Print and shaded views of the part. All mm, measured from the part's lowest x, y and z. A direction names the side the tool comes from. Coordinates: 2 decimals unless noted, no trailing zeros. Loops run counter-clockwise (first coordinate to the right, second up) from the corner with the lowest first, then second, coordinate; pieces in that order, holes last. Notation, with made-up numbers: M 60,1.25 L 79,1.25 A14 cw 79,8.25 Z; hole C 72,-7.75 d4. An arc over 180 degrees is marked long. Use a Markdown table: item, result. Add a question column.
1) Pin check, flat tips, straight feed: pin 1 Ø3 at (y, z) = (8.5, 92) entering from -X; pin 2 Ø3 at (y, z) = (9.5, 87.5) entering from -X; pin 3 Ø6 at (x, z) = (7, 98) entering from -Y. Stop position of each tip, or through.
2) Band-saw the part on C-C (z = 15). List the corners of the cut face in (x, y) (1 decimal).
3) Band-saw the part on A-A (x = 6.75). List the corners of the cut face in (y, z), plus the area to 3 significant figures.
4) Band-saw the part on B-B (y = 8.5). List the corners of the cut face in (x, z) (1 decimal).
5) Wall check: probe 1 along Z at (x, y) = (3.25, 1.75); probe 2 along Y at (x, z) = (7, 19.5); probe 3 along X at (y, z) = (8.25, 102.5). Give the ranges that are in metal, low to high. Write a range as from..to.
6) Band-saw the part on D-D (x = 12.5). List the corners of the cut face in (y, z), plus the area to 3 significant figures.
7) Tool access for the marked faces 1 and 2: list every direction of +Z, -Z, +X, -X, +Y, -Y with a clear straight run to the whole face (end or side of a thin tool).
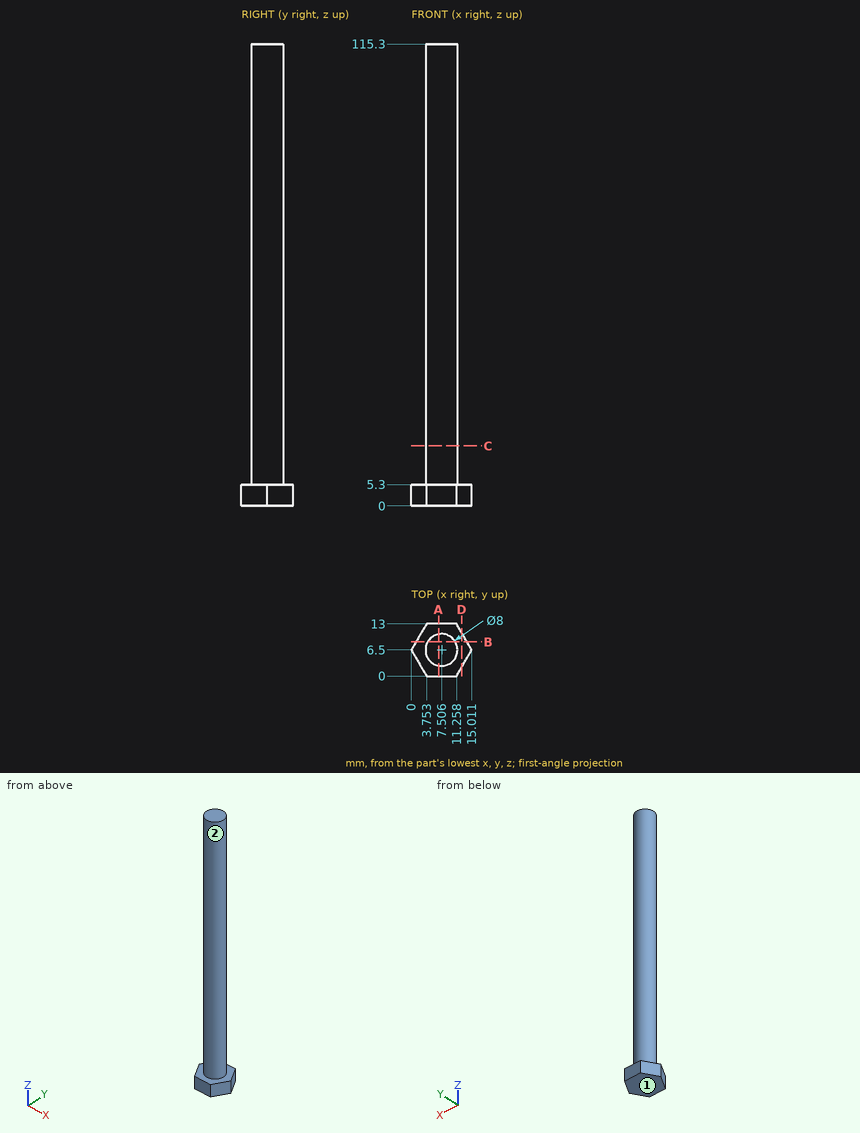
Entries:
| question | item | result |
|---|---|---|
| 1 | pin 1 | x = 3.54 |
| 1 | pin 2 | x = 3.8 |
| 1 | pin 3 | y = 2.5 |
| 2 | outline | C 7.5,6.5 d8 |
| 3 | outline | M 0,0 L 13,0 L 13,5.3 L 10.43,5.3 L 10.43,115.3 L 2.57,115.3 L 2.57,5.3 L 0,5.3 Z |
| 3 | area | 933 mm2 |
| 4 | outline | M 1.2,0 L 13.9,0 L 13.9,5.3 L 11,5.3 L 11,115.3 L 4,115.3 L 4,5.3 L 1.2,5.3 Z |
| 5 | probe 1 | 0..5.3 |
| 5 | probe 2 | 2.53..10.47 |
| 5 | probe 3 | 3.91..11.1 |
| 6 | outline | M 2.15,0 L 10.85,0 L 10.85,5.3 L 2.15,5.3 Z |
| 6 | area | 46.1 mm2 |
| 7 | face 1 | -Z, +X, -X, +Y, -Y |
| 7 | face 2 | +Z |
